```python
from build123d import *

# Parameters (mm, degrees)
CORTAR_EXTRUIR1_DEPTH      = 15
CORTAR_EXTRUIR1_DEPTH_BACK = 10
CROQUIS2_W                 = 7.74823864
CROQUIS2_H                 = 16.99585586
CROQUIS4_R                 = 5
SALIENTE_EXTRUIR2_DEPTH    = 20
CORTAR_EXTRUIR2_DEPTH      = 2
CORTAR_EXTRUIR2_DEPTH_BACK = 2
CROQUIS6_W                 = 2
CROQUIS6_H                 = 2.5


with BuildPart() as part:
    # Croquis1 → Revolución2 (revolve)
    with BuildSketch(Plane.XY, mode=Mode.PRIVATE) as revoluci_n2_sk:
        with BuildLine():
            Line((0, 9), (0, -11))
            Line((0, -11), (0, -12))
            Line((0, -12), (0, -15))
            Line((0, -15), (2, -15))
            Line((2, -15), (2, -10))
            Line((2, -10), (3.455214016, -10))
            Line((3.455214016, -10), (3.455214016, -9))
            Line((3.455214016, -9), (10.723805295, -9))
            ThreePointArc((10.723805295, -9), (14, 0), (10.723805295, 9))
            Line((10.723805295, 9), (3.47289893, 9))
            Line((3.47289893, 9), (3.47289893, 10))
            Line((3.47289893, 10), (2, 10))
            Line((2, 10), (2, 13))
            Line((2, 13), (0, 13))
            Line((0, 13), (0, 10))
            Line((0, 10), (0, 9))
        make_face()
    revolve(revoluci_n2_sk.sketch.rotate(Axis((0, 9, 0), (0, -1, 0)), 90), axis=Axis((0, 9, 0), (0, -1, 0)))

    # Croquis2 → Cortar-Extruir1 (cut, two sides: drawn at the far end of the back side and taken through both)
    with BuildSketch(Plane(origin=(0, 0, 0), x_dir=(0, 0, -1), z_dir=(1, 0, 0)).offset(-CORTAR_EXTRUIR1_DEPTH_BACK)):
        with Locations((-15, 0)):
            Rectangle(CROQUIS2_W, CROQUIS2_H)
    extrude(amount=CORTAR_EXTRUIR1_DEPTH + CORTAR_EXTRUIR1_DEPTH_BACK, mode=Mode.SUBTRACT)

    # Croquis4 → Saliente-Extruir2 (add)
    with BuildSketch(Plane.XY.offset(11.12588068)):
        Circle(CROQUIS4_R)
    extrude(amount=SALIENTE_EXTRUIR2_DEPTH)

    # Croquis6 → Cortar-Extruir2 (cut, two sides: drawn at the far end of the back side and taken through both)
    with BuildSketch(Plane.XY.offset(-CORTAR_EXTRUIR2_DEPTH_BACK)):
        with Locations((0, 11.75)):
            Rectangle(CROQUIS6_W, CROQUIS6_H)
    extrude(amount=CORTAR_EXTRUIR2_DEPTH + CORTAR_EXTRUIR2_DEPTH_BACK, mode=Mode.SUBTRACT)


solid = part.part
```
Build history of the part. All positions in model axes, mm. A direction names the side the tool comes from. Round coordinates to 2 decimals unless told otherwise and drop trailing zeros. Loops run counter-clockwise (first coordinate to the right, second up) from the corner with the lowest first, then second, coordinate; pieces in that order, holes last.
Item 1: Which spindle directions (+Z, -Z, +X, -X, +Y, -Y) get a long thin tool onto all of the face, cutting with end or side? Do faces 4 (the face through (4, 4, 11.126)), 5 (the face through (-3, -9, 3)), 6 (the face through (-3, 9, -3)), 7 (the face through (-1, 12, 0)). Say none if no direction does.
Item 2: Saw through at D-D (x = 6.75). List the corners of the cut face in (y, z).
Item 3: Saw through at C-C (y = 0). List the corners of the cut face in (x, z).
Item 4: Saw through at A-A (z = 0). List the corners of the cut face in (x, y).
Item 5: Saw through at B-B (x = 0). List the corners of the cut face in (y, z).
Item 6: Pin check, flat tips, straight feed: P1, Ø1, axis at x = 1.5, y = -6.5, coming from the +Z side; P2, Ø2, axis at y = 4.5, z = 13.5, coming from the +X side; P3, Ø7.5, axis at x = 0, z = 0, coming from the +Y side; P4, Ø1.5, axis at y = 7.5, z = 2.5, coming from the -X side. Stop position of each tip, or through.
Item 7: Drill centre lines: line 1 along Y through (x, z) = (10, -1); line 2 along X through (y, z) = (1, 16); line 3 along Z through (x, y) = (11.75, -5.5). Where is each one in solid material? Low to high.
Item 8: Two-plate mould, pull along X, no slides. Class faces 1 (the face through (0, -15, 0)), 2 (the face through (-1.043, 9.507, 3.313)), 3 (the face through (1, 12, 0)): released by +X, released by -X, zero draft, split by the parting line, or undercut.
Worked answers:
1. face 4: +Z
1. face 5: -Y
1. face 6: +Y
1. face 7: +Z, -Z, +Y
2. outline: (-9, -8.33) arc R12.27 ccw to (9, -8.33) - (9, 8.33) arc R12.27 ccw to (5.16, 11.13) - (-5.16, 11.13) arc R12.27 ccw to (-9, 8.33) - close
3. outline: (-8.5, 11.13) arc R14 ccw (long way) to (8.5, 11.13) - (5, 11.13) - (5, 31.13) - (-5, 31.13) - (-5, 11.13) - close
4. outline: (-10.72, -9) - (-3.46, -9) - (-3.46, -10) - (-2, -10) - (-2, -15) - (2, -15) - (2, -10) - (3.46, -10) - (3.46, -9) - (10.72, -9) arc R14 ccw to (10.72, 9) - (3.47, 9) - (3.47, 10) - (2, 10) - (2, 13) - (1, 13) - (1, 10.5) - (-1, 10.5) - (-1, 13) - (-2, 13) - (-2, 10) - (-3.47, 10) - (-3.47, 9) - (-10.72, 9) arc R14 ccw to start
5. outline: (-15, -2) - (-10, -2) - (-10, -3.46) - (-9, -3.46) - (-9, -10.72) arc R14 ccw to (9, -10.72) - (9, -3.47) - (10, -3.47) - (10, -2) - (10.5, -2) - (10.5, 2) - (10, 2) - (10, 3.47) - (9, 3.47) - (9, 10.72) arc R14 ccw to (8.5, 11.13) - (5, 11.13) - (5, 31.13) - (-5, 31.13) - (-5, 11.13) - (-8.5, 11.13) arc R14 ccw to (-9, 10.72) - (-9, 3.46) - (-10, 3.46) - (-10, 2) - (-15, 2) - close
6. P1: stops at z = 11.13
6. P2: stops at x = 3.57
6. P3: stops at y = 13
6. P4: stops at x = -12.03
7. line 1: y = -9 to 9
7. line 2: x = -4.9 to 4.9
7. line 3: z = -5.26 to 5.26
8. face 1: zero draft
8. face 2: split by the parting line
8. face 3: undercut
